```python
from build123d import *

# Parameters (mm, degrees)
SKETCH_1_R                         = 2.25
SM_BASE_FLANGE_1_DEPTH             = 1.5
SM_EDGE_FLANGE_1_STRIP_W           = 6.2
SM_EDGE_FLANGE_1_STRIP_H           = 1.5
SM_EDGE_FLANGE_1_STRIP_CUT_DEPTH   = 115
SM_EDGE_FLANGE_1_STRIP_2_W         = 6.2
SM_EDGE_FLANGE_1_STRIP_2_H         = 1.5
SM_EDGE_FLANGE_1_STRIP_CUT_2_DEPTH = 115
SM_EDGE_FLANGE_1_DEPTH             = 115
SM_EDGE_FLANGE_1_BEND_DEPTH        = 115
SM_START                           = 471.682547587
SM_EDGE_FLANGE_2_DEPTH             = 1180
SM_EDGE_FLANGE_2_2_DEPTH           = 1.6
SM_START_2                         = 1650.082547587
SM_EDGE_FLANGE_2_3_DEPTH           = 1.6
SM_START_3                         = 473.282547587
SM_EDGE_FLANGE_2_4_DEPTH           = 1176.8
SKETCH_15_R                        = 5
CUT_EXTRUDE_1_DEPTH                = 10


# Read off the part's stored shape, not the designer's step: 边线-法兰2
# Sheet-metal steps are written as plain solids
with BuildPart() as part:
    # Sketch 1 → 基体-法兰1 (new body)
    with BuildSketch(Plane.XY):
        with BuildLine():
            Line((471.682547587, -1331.896552128), (473.182547587, -1331.896552128))
            Line((473.182547587, -1331.896552128), (473.919147587, -1331.896552128))
            Line((473.919147587, -1331.896552128), (599.182547587, -1331.896552128))
            Line((599.182547587, -1331.896552128), (599.182547587, -1318.896552128))
            ThreePointArc((599.182547587, -1318.896552128), (661.682547587, -1256.396552128), (724.182547587, -1318.896552128))
            Line((724.182547587, -1318.896552128), (724.182547587, -1331.896552128))
            Line((724.182547587, -1331.896552128), (1399.182547587, -1331.896552128))
            Line((1399.182547587, -1331.896552128), (1399.182547587, -1318.896552128))
            ThreePointArc((1399.182547587, -1318.896552128), (1461.682547587, -1256.396552128), (1524.182547587, -1318.896552128))
            Line((1524.182547587, -1318.896552128), (1524.182547587, -1331.896552128))
            Line((1524.182547587, -1331.896552128), (1649.445947587, -1331.896552128))
            Line((1649.445947587, -1331.896552128), (1650.182547587, -1331.896552128))
            Line((1650.182547587, -1331.896552128), (1651.682547587, -1331.896552128))
            Line((1651.682547587, -1331.896552128), (1651.682547587, -1216.896552128))
            Line((1651.682547587, -1216.896552128), (471.682547587, -1216.896552128))
            Line((471.682547587, -1216.896552128), (471.682547587, -1331.896552128))
        make_face()
        with Locations((801.682547587, -1274.396552128)):
            Circle(SKETCH_1_R, mode=Mode.SUBTRACT)
        with Locations((1321.682547587, -1274.396552128)):
            Circle(SKETCH_1_R, mode=Mode.SUBTRACT)
        with Locations((506.682547587, -1274.396552128)):
            Circle(SKETCH_1_R, mode=Mode.SUBTRACT)
        with Locations((1061.682547587, -1274.396552128)):
            Circle(SKETCH_1_R, mode=Mode.SUBTRACT)
        with Locations((1616.682547587, -1274.396552128)):
            Circle(SKETCH_1_R, mode=Mode.SUBTRACT)
    extrude(amount=-SM_BASE_FLANGE_1_DEPTH)

    # 边线-法兰1 strip (across the edge) → 边线-法兰1 strip cut (cut)
    with BuildSketch(Plane(origin=(1651.682547587, -1331.896552128, 0), x_dir=(-1, 0, 0), z_dir=(0, 1, 0))):
        with Locations((-1.5, -0.75)):
            Rectangle(SM_EDGE_FLANGE_1_STRIP_W, SM_EDGE_FLANGE_1_STRIP_H)
    extrude(amount=SM_EDGE_FLANGE_1_STRIP_CUT_DEPTH, mode=Mode.SUBTRACT)

    # 边线-法兰1 strip 2 (across the edge) → 边线-法兰1 strip cut 2 (cut)
    with BuildSketch(Plane(origin=(471.682547587, -1216.896552128, 0), x_dir=(1, 0, 0), z_dir=(0, -1, 0))):
        with Locations((-1.5, -0.75)):
            Rectangle(SM_EDGE_FLANGE_1_STRIP_2_W, SM_EDGE_FLANGE_1_STRIP_2_H)
    extrude(amount=SM_EDGE_FLANGE_1_STRIP_CUT_2_DEPTH, mode=Mode.SUBTRACT)

    # 边线-法兰1 section (across the edge) → 边线-法兰1 (add)
    with BuildSketch(Plane(origin=(1651.682547587, -1331.896552128, 0), x_dir=(-1, 0, 0), z_dir=(0, 1, 0))):
        with BuildLine():
            Line((0, 0.1), (0, 58.5))
            Line((0, 58.5), (1.5, 58.5))
            Line((1.5, 58.5), (1.5, 0.1))
            ThreePointArc((1.5, 0.1), (1.529289322, 0.029289322), (1.6, 0))
            Line((1.6, 0), (1.6, -1.5))
            ThreePointArc((1.6, -1.5), (0.46862915, -1.03137085), (0, 0.1))
        make_face()
    extrude(amount=SM_EDGE_FLANGE_1_DEPTH)

    # 边线-法兰1 section 2 (across the edge) → 边线-法兰1 bend (add)
    with BuildSketch(Plane(origin=(471.682547587, -1216.896552128, 0), x_dir=(1, 0, 0), z_dir=(0, -1, 0))):
        with BuildLine():
            Line((0, 0.1), (0, 58.5))
            Line((0, 58.5), (1.5, 58.5))
            Line((1.5, 58.5), (1.5, 0.1))
            ThreePointArc((1.5, 0.1), (1.529289322, 0.029289322), (1.6, 0))
            Line((1.6, 0), (1.6, -1.5))
            ThreePointArc((1.6, -1.5), (0.46862915, -1.03137085), (0, 0.1))
        make_face()
    extrude(amount=SM_EDGE_FLANGE_1_BEND_DEPTH)

    # 边线-法兰2 outline → 边线-法兰2 (cut)
    with BuildSketch(Plane.YZ.offset(SM_START)):
        with BuildLine():
            Line((-1218.396552128, 0.1), (-1218.496552128, 0.1))
            Line((-1218.496552128, 0.1), (-1218.496552128, 0))
            ThreePointArc((-1218.496552128, 0), (-1218.42584145, 0.029289322), (-1218.396552128, 0.1))
        make_face()
        with BuildLine():
            ThreePointArc((-1216.896552128, 0.1), (-1217.365181278, -1.03137085), (-1218.496552128, -1.5))
            Line((-1218.496552128, -1.5), (-1216.896552128, -1.5))
            Line((-1216.896552128, -1.5), (-1216.896552128, 0.1))
        make_face()
    extrude(amount=SM_EDGE_FLANGE_2_DEPTH, mode=Mode.SUBTRACT)

    # Sm Edge Flange 2 2 outline → Sm Edge Flange 2 2 (cut)
    with BuildSketch(Plane.YZ.offset(SM_START)):
        with BuildLine():
            Line((-1216.896552128, 0.1), (-1218.396552128, 0.1))
            ThreePointArc((-1218.396552128, 0.1), (-1218.42584145, 0.029289322), (-1218.496552128, 0))
            Line((-1218.496552128, 0), (-1218.496552128, -1.5))
            ThreePointArc((-1218.496552128, -1.5), (-1217.365181278, -1.03137085), (-1216.896552128, 0.1))
        make_face()
    extrude(amount=SM_EDGE_FLANGE_2_2_DEPTH, mode=Mode.SUBTRACT)

    # Sm Edge Flange 2 3 outline → Sm Edge Flange 2 3 (cut)
    with BuildSketch(Plane.YZ.offset(SM_START_2)):
        with BuildLine():
            Line((-1216.896552128, 0.1), (-1218.396552128, 0.1))
            ThreePointArc((-1218.396552128, 0.1), (-1218.42584145, 0.029289322), (-1218.496552128, 0))
            Line((-1218.496552128, 0), (-1218.496552128, -1.5))
            ThreePointArc((-1218.496552128, -1.5), (-1217.365181278, -1.03137085), (-1216.896552128, 0.1))
        make_face()
    extrude(amount=SM_EDGE_FLANGE_2_3_DEPTH, mode=Mode.SUBTRACT)

    # Sm Edge Flange 2 4 outline → Sm Edge Flange 2 4 (add)
    with BuildSketch(Plane.YZ.offset(SM_START_3)):
        with BuildLine():
            Line((-1218.396552128, 58.5), (-1218.396552128, 0.1))
            ThreePointArc((-1218.396552128, 0.1), (-1218.42584145, 0.029289322), (-1218.496552128, 0))
            Line((-1218.496552128, 0), (-1216.899680186, 0))
            ThreePointArc((-1216.899680186, 0), (-1216.897334334, 0.049975544), (-1216.896552128, 0.1))
            Line((-1216.896552128, 0.1), (-1216.896552128, 58.5))
            Line((-1216.896552128, 58.5), (-1218.396552128, 58.5))
        make_face()
    extrude(amount=SM_EDGE_FLANGE_2_4_DEPTH)

    # 草图15 → 切除-拉伸1 (cut)
    with BuildSketch(Plane(origin=(0, -1216.896552128, 0), x_dir=(1, 0, 0), z_dir=(0, 1, 0))):
        with Locations(Location((619.182547587, -48.5, 0), (0, 0, 270))):
            Circle(SKETCH_15_R)
        with Locations(Location((584.182547587, -48.5, 0), (0, 0, 270))):
            Circle(SKETCH_15_R)
        with Locations(Location((1079.182547587, -48.5, 0), (0, 0, 270))):
            Circle(SKETCH_15_R)
        with Locations(Location((1044.182547587, -48.5, 0), (0, 0, 270))):
            Circle(SKETCH_15_R)
        with Locations(Location((1504.182547587, -48.5, 0), (0, 0, 270))):
            Circle(SKETCH_15_R)
        with Locations(Location((1539.182547587, -48.5, 0), (0, 0, 270))):
            Circle(SKETCH_15_R)
    extrude(amount=-CUT_EXTRUDE_1_DEPTH, mode=Mode.SUBTRACT)


solid = part.part
```
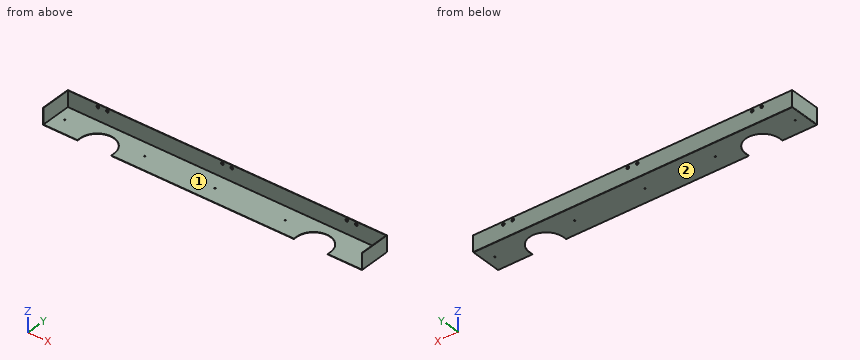
Geometry: final body of the model. Coordinates: model frame, mm. Face numbers are marked on the shaded views. A direction names the side the tool comes from. Give positions to 0.01 mm unless a question says otherwise; leave off trailing zeros. Write each loop counter-clockwise with the first axis right and the second up, starting at its lowest first coordinate (ties: lowest second). Pieces come first, ordered by that corner, then holes.
1. Reachability of the marked faces 1 and 2 from +Z, -Z, +X, -X, +Y, -Y: full face, straight path, thin tool, end or side. Return the list, or none.
2. Line query: probe 1 along X at (y, z) = (-1308, 38.5); probe 2 along Y at (x, z) = (868, 7); probe 3 along Z at (x, y) = (1562.5, -1308). Output: solid intervals per line, ascending.
3. Section query B-B, the plane y = -1234.5. Return loops of the section in (x, z).
4. Section query C-C, the plane x = 1344. Return loops of the section in (y, z).
5. Pin query (flat end, axial travel): P1, Ø4, axis at x = 603, y = -1236.5, coming from the +Z side; P2, Ø16, axis at x = 619.18, z = 48.5, coming from the +Y side; P3, Ø2, axis at x = 1172, z = 37, coming from the -Y side; P4, Ø0.5, axis at x = 472, z = -0.5, coming from the +Y side. Return the tip coordinate at first contact, or that it passes through.
6. Section query A-A, the plane z = 20. Return loops of the section in (x, y).
Computed:
1. face 1: +Z, -Y
1. face 2: -Z, +X, -X, +Y, -Y
2. probe 1: x = 471.68 to 473.18, 1650.18 to 1651.68
2. probe 2: y = -1218.4 to -1216.9
2. probe 3: z = -1.5 to 0
3. outline: (471.68, 0.1) arc R1.6 ccw to (473.28, -1.5) - (1650.08, -1.5) arc R1.6 ccw to (1651.68, 0.1) - (1651.68, 58.5) - (1650.18, 58.5) - (1650.18, 0.1) arc R0.1 cw to (1650.08, 0) - (473.28, 0) arc R0.1 cw to (473.18, 0.1) - (473.18, 58.5) - (471.68, 58.5) - close
4. outline: (-1331.9, -1.5) - (-1218.5, -1.5) arc R1.6 ccw to (-1216.9, 0.1) - (-1216.9, 58.5) - (-1218.4, 58.5) - (-1218.4, 0.1) arc R0.1 cw to (-1218.5, 0) - (-1331.9, 0) - close
5. P1: stops at z = 0
5. P2: stops at y = -1216.9
5. P3: stops at y = -1218.4
5. P4: stops at y = -1218.5
6. outline: (471.68, -1331.9) - (473.18, -1331.9) - (473.18, -1216.9) - (471.68, -1216.9) - close; (473.28, -1218.4) - (1650.08, -1218.4) - (1650.08, -1216.9) - (473.28, -1216.9) - close; (1650.18, -1331.9) - (1651.68, -1331.9) - (1651.68, -1216.9) - (1650.18, -1216.9) - close
